from build123d import *

# Parameters (mm, degrees)
F3_DEPTH = 101.6
F4_DEPTH = 282.663077116
F5_R     = 3.175
F6_DEPTH = 127
F7_DEPTH = 6.35
F8_W     = 50.8
F8_H     = 50.8
F8_H_2   = 25.4
F9_DEPTH = 127
F10_R    = 12.7


with BuildPart() as f3:
    # F0 (on Front) → F3 (new body)
    with BuildSketch(Plane.XZ):
        with BuildLine():
            Line((50.8, -85.7884685198), (50.8, 0))
            ThreePointArc((50.8, 0), (0, -50.8), (-50.8, 0))
            Line((-50.8, 0), (-50.8, -85.7884685198))
            Line((-50.8, -85.7884685198), (50.8, -85.7884685198))
        make_face()
        with BuildLine():
            ThreePointArc((-50.8, 0), (0, -50.8), (50.8, 0))
            ThreePointArc((50.8, 0), (0, 50.8), (-50.8, 0))
        make_face()
    extrude(amount=F3_DEPTH)

    # F2 (on face) + F1 (on Front) → F4 (cut)
    with BuildSketch(Plane.XZ):
        with BuildLine():
            Line((-1.1809319258, -85.7884685198), (1.1809319258, -85.7884685198))
            Line((1.1809319258, -85.7884685198), (1.1809319258, -50.786271765))
            ThreePointArc((1.1809319258, -50.786271765), (0, -50.8), (-1.1809319258, -50.786271765))
            Line((-1.1809319258, -50.786271765), (-1.1809319258, -85.7884685198))
        make_face()
        with BuildLine():
            ThreePointArc((-1.1809319258, -50.786271765), (0, -50.8), (1.1809319258, -50.786271765))
            Line((1.1809319258, -50.786271765), (1.1809319258, 14.9626284838))
            Line((1.1809319258, 14.9626284838), (-1.1809319258, 14.9626284838))
            Line((-1.1809319258, 14.9626284838), (-1.1809319258, -50.786271765))
        make_face()
    with BuildSketch(Plane.XZ):
        Polygon((35.9210244843, 0), (0, 35.9210244843), (-35.9210244843, 0), (0, -35.9210244843), align=None)
    extrude(amount=F4_DEPTH, mode=Mode.SUBTRACT)

    # F5 (on face) → F6 (cut)
    with BuildSketch(Plane.YZ.offset(50.8)):
        with Locations((-42.7350864422, -42.1568825841)):
            Circle(F5_R)
        with Locations((-61.7602499746, -42.1568825841)):
            Circle(F5_R)
    extrude(amount=-F6_DEPTH, mode=Mode.SUBTRACT)

    # F5 (on face) → F7 (cut)
    with BuildSketch(Plane.YZ.offset(50.8)):
        Polygon((-62.336745475, -47.4765820931), (-57.4415028095, -45.3159920871), (-56.8650073091, -39.9962925781), (-61.1837544742, -36.8371830751), (-66.0789971397, -38.9977730811), (-66.6554926401, -44.3174725901), align=None)
        with Locations((-61.7602499746, -42.1568825841)):
            Circle(F5_R, mode=Mode.SUBTRACT)
        Polygon((-43.2069172048, -47.486893887), (-38.3550766327, -45.2305056623), (-37.88324587, -39.9004943594), (-42.2632556795, -36.8268712812), (-47.1150962516, -39.0832595059), (-47.5869270143, -44.4132708088), align=None)
        with Locations((-42.7350864422, -42.1568825841)):
            Circle(F5_R, mode=Mode.SUBTRACT)
    extrude(amount=-F7_DEPTH, mode=Mode.SUBTRACT)

    # F8 (on face) → F9 (cut)
    with BuildSketch(Plane.YZ.offset(50.8)):
        with Locations((-50.8, -85.7884685198)):
            Rectangle(F8_W, F8_H)
        with Locations((-50.8, -73.0884685198)):
            Rectangle(F8_W, F8_H_2)
    extrude(amount=-F9_DEPTH, mode=Mode.SUBTRACT)

    # F10
    f10_edges = [f3.edges().sort_by_distance(p)[0] for p in [
        (0, -101.6, 50.8),
        (50.8, -101.6, -42.894234),
        (0, 0, 50.8),
        (50.8, 0, -42.894234),
        (-50.8, 0, -42.894234),
        (-50.8, -101.6, -42.894234),
    ]]
    fillet(f10_edges, radius=F10_R)


solid = f3.part
Geometry check sheet. Reference: the model listing, model coordinates, mm. A direction names the side the tool comes from. Give positions to 0.01 mm unless a question says otherwise; leave off trailing zeros. Order: outer loops, then holes, each group sorted by start corner. A loop starts at its lowest first (then second) coordinate and runs counter-clockwise, first axis right, second up. Notation, with made-up numbers: M 60,5 L 66,5 A24 ccw 66,44 Z; hole C 69,-36 d6. An arc over 180 degrees is marked long. Use a Markdown table: item, result.
Item 1: Section check A-A (y = -16). Record the cut outline in (x, z), and give its area (3 significant figures).
Answers follow:
| item | result |
|---|---|
| outline | M -50.8,-85.79 L -1.18,-85.79 L -1.18,-34.74 L -35.92,0 L 0,35.92 L 35.92,0 L 1.18,-34.74 L 1.18,-85.79 L 50.8,-85.79 L 50.8,0 A50.8 ccw -50.8,0 Z |
| area | 10,100 mm2 |
Item 2: Material ranges on line 1 along Y through (x, z) = (-2, -73); line 2 along X through (y, z) = (-51, -43.5); line 3 along Y through (x, z) = (44, -71.5), recorded low to high.
Answers follow:
| item | result |
|---|---|
| line 1 | y = -101.6 to -76.2, -25.4 to 0 |
| line 2 | x = -50.8 to -1.18, 1.18 to 50.8 |
| line 3 | y = -100.15 to -76.2, -25.4 to -1.45 |
Item 3: Draft check along Z on faces 4 (the flat face through (26, -89, -85.788)), 5 (the cylindrical face through (-46.98, -3.62, -43.49)), 6 (the flat face through (47.67, -58.99, -38.44)). Enter one of: +Z half, -Z half, draft (parallel to the pull), parting line (faces both ways), or undercut.
Answers follow:
| item | result |
|---|---|
| face 4 | -Z half |
| face 5 | draft |
| face 6 | undercut |
Item 4: Tool access check on faces 1 (the flat face through (47.669, -63.597, -37.902)), 2 (the flat face through (18.31, -50.09, -17.61)), 3 (the flat face through (26, -76.2, -73)). Record the directions out of +Z, -Z, +X, -X, +Y, -Y that give a thin tool (end or side, any length) a straight path to the whole face; none if there is none.
Answers follow:
| item | result |
|---|---|
| face 1 | +X |
| face 2 | +Y, -Y |
| face 3 | -Z, +X, -X |
Item 5: Depth check by flat-ended pin: P1, Ø8, axis at x = 28.5, y = -49.5, coming from the +Z side; P2, Ø5, axis at y = -42.5, z = -43.5, coming from the +X side; P3, Ø3, axis at y = -47.5, z = 6, coming from the +X side. Enter the tip coordinate at first touch or a pass-through.
Answers follow:
| item | result |
|---|---|
| P1 | stops at z = 44.5 |
| P2 | stops at x = 44.45 |
| P3 | stops at x = 50.6 |
Item 6: Section check D-D (y = -34). Record the cut outline in (x, z), and give its area (3 significant figures).
Answers follow:
| item | result |
|---|---|
| outline | M -50.8,-60.39 L -1.18,-60.39 L -1.18,-34.74 L -35.92,0 L 0,35.92 L 35.92,0 L 1.18,-34.74 L 1.18,-60.39 L 50.8,-60.39 L 50.8,0 A50.8 ccw -50.8,0 Z |
| area | 7,550 mm2 |
Item 7: Section check B-B (x = -5). State how many separate pieces and enclosed holes the cut face has, and give its area (3 significant figures).
Answers follow:
| item | result |
|---|---|
| separate pieces | 2 |
| enclosed holes | 2 |
| area | 6,150 mm2 |
